```python
from build123d import *

# Parameters (mm, degrees)
BOSS_EXTRUDE1_DEPTH     = 1
SKETCH2_R               = 0.5
BOSS_EXTRUDE2_DEPTH     = 7
SKETCH4_W               = 11
SKETCH4_H               = 4
CUT_EXTRUDE1_DEPTH      = 1
CUT_EXTRUDE1_DEPTH_BACK = 9
CHAMFER2_SIZE           = 0.1


with BuildPart() as part:
    # Sketch1 → Boss-Extrude1 (new body)
    with BuildSketch(Plane(origin=(0, 0, 0), x_dir=(1, 0, 0), z_dir=(0, 1, 0))):
        with BuildLine():
            Line((-16, -6.5), (16, -6.5))
            ThreePointArc((16, -6.5), (16.707106781, -6.207106781), (17, -5.5))
            Line((17, -5.5), (17, 5.5))
            ThreePointArc((17, 5.5), (16.707106781, 6.207106781), (16, 6.5))
            Line((16, 6.5), (-16, 6.5))
            ThreePointArc((-16, 6.5), (-16.707106781, 6.207106781), (-17, 5.5))
            Line((-17, 5.5), (-17, -5.5))
            ThreePointArc((-17, -5.5), (-16.707106781, -6.207106781), (-16, -6.5))
        make_face()
    extrude(amount=BOSS_EXTRUDE1_DEPTH)

    # Sketch2 → Boss-Extrude2 (add)
    with BuildSketch(Plane.XZ):
        with Locations((-15.25, 4.75)):
            Circle(SKETCH2_R)
        with Locations((-15.25, -4.75)):
            Circle(SKETCH2_R)
        with Locations((8.25, -4.75)):
            Circle(SKETCH2_R)
        with Locations((8.25, 4.75)):
            Circle(SKETCH2_R)
    extrude(amount=BOSS_EXTRUDE2_DEPTH)

    # Sketch4 → Cut-Extrude1 (cut, two sides)
    with BuildSketch(Plane(origin=(0, 1, 0), x_dir=(1, 0, 0), z_dir=(0, 1, 0))) as cut_extrude1_sk:
        with Locations((-3.5, 0)):
            Rectangle(SKETCH4_W, SKETCH4_H)
    extrude(amount=CUT_EXTRUDE1_DEPTH, mode=Mode.SUBTRACT)
    extrude(cut_extrude1_sk.sketch, amount=-CUT_EXTRUDE1_DEPTH_BACK, mode=Mode.SUBTRACT)

    # Chamfer2
    chamfer2_edges = [part.edges().sort_by_distance(p)[0] for p in [
        (-15.75, -7, 4.75),
        (7.75, -7, 4.75),
        (7.75, -7, -4.75),
        (-15.75, -7, -4.75),
    ]]
    chamfer(chamfer2_edges, length=CHAMFER2_SIZE)


solid = part.part
```
Could you check a few things on this model? Use its own coordinates, in mm. A direction names the side the tool comes from. Round coordinates to 2 decimals unless told otherwise and drop trailing zeros. Loops run counter-clockwise (first coordinate to the right, second up) from the corner with the lowest first, then second, coordinate; pieces in that order, holes last. Notation, with made-up numbers: (-15, 60.25) - (37, 60.25) arc R28 cw to (37, 97.25) - close; hole circle Ø2 at (19, 3.5). An arc over 180 degrees is marked (long way). Answer in a Markdown table with one row per item. Add a question column.
(1) For faces 4 (the face through (8.727, -3.402, 4.9)), 5 (the face through (2, 0.5, 0)), 6 (the face through (-16.715, 0.493, 6.199)), which set-ups out of +Z, -Z, +X, -X, +Y, -Y let a thin tool reach every point of the face, with its end or its side?
(2) I'm going to push a flat-ended pin straight in: pin 1 (6 mm diameter, centred on x = -3, z = 0.5, fed in from -Y). Where does the tip first touch, or does it pass through?
(3) If we mould it in two halves opening along X, with no side actions, what happens to faces 1 (the face through (0.2, 0.5, -6.5)), 2 (the face through (-16.699, 0.493, -6.215)), 3 (the face through (-15.315, -3.402, 5.246))? For each: pulls with the +X half, pulls with the -X half, needs draft (parallel to the pull), parting line crosses it, or undercut.
(4) If we section it at D-D (z = 4.75): Please give me the cut outline in (x, y).
(5) If we section it at B-B (z = -1.5): Please give me the cut outline in (x, y), plus the area to 3 significant figures.
(6) If we section it at C-C (y = -2.25): Please give me the cut outline in (x, z).
(7) I need wall thicknesses on line 1 along Y through (x, z) = (-1, -3.5); line 2 along X through (y, z) = (-4.75, 4.5); line 3 along Z through (x, y) = (-15.5, -5). Which ranges of each line are inside material? Lowest first, please.
(8) If we section it at A-A (x = -7): Please give me the cut outline in (y, z), plus the area to 3 significant figures.
Model answer:
| question | item | result |
|---|---|---|
| 1 | face 4 | -Y |
| 1 | face 5 | +Y, -Y |
| 1 | face 6 | +Z, -X, +Y, -Y |
| 2 | pin 1 | stops at y = 0 |
| 3 | face 1 | needs draft |
| 3 | face 2 | pulls with the -X half |
| 3 | face 3 | undercut |
| 4 | outline | (-17, 0) - (-15.75, 0) - (-15.75, -6.9) - (-15.65, -7) - (-14.85, -7) - (-14.75, -6.9) - (-14.75, 0) - (7.75, 0) - (7.75, -6.9) - (7.85, -7) - (8.65, -7) - (8.75, -6.9) - (8.75, 0) - (17, 0) - (17, 1) - (-17, 1) - close |
| 5 | outline | (-17, 0) - (-9, 0) - (-9, 1) - (-17, 1) - close; (2, 0) - (17, 0) - (17, 1) - (2, 1) - close |
| 5 | area | 23.0 mm² |
| 6 | outline | circle Ø1 at (-15.25, -4.75); circle Ø1 at (-15.25, 4.75); circle Ø1 at (8.25, -4.75); circle Ø1 at (8.25, 4.75) |
| 7 | line 1 | y = 0 to 1 |
| 7 | line 2 | x = -15.68 to -14.82, 7.82 to 8.68 |
| 7 | line 3 | z = -5.18 to -4.32, 4.32 to 5.18 |
| 8 | outline | (0, -6.5) - (1, -6.5) - (1, -2) - (0, -2) - close; (0, 2) - (1, 2) - (1, 6.5) - (0, 6.5) - close |
| 8 | area | 9.00 mm² |
